```python
from build123d import *

# Parameters (mm, degrees)
BOSS_EXTRU_1_DEPTH           = 3
ESQUISSE26_W                 = 21
ESQUISSE26_H                 = 42
ENL_V_MAT_EXTRU_1_DEPTH      = 4
ESQUISSE21_W                 = 11.4
ESQUISSE21_H                 = 11.4
ENL_V_MAT_EXTRU_3_DEPTH      = 4
D_GAGEMENT_M32_D             = 3.4
D_GAGEMENT_M33_D             = 3.4
ENL_V_MAT_EXTRU_4_DEPTH      = 10
ENL_V_MAT_EXTRU_4_DEPTH_BACK = 4
D_GAGEMENT_M41_D             = 4.5
ESQUISSE40_W                 = 13
ESQUISSE40_H                 = 13
ENL_V_MAT_EXTRU_5_DEPTH      = 4


with BuildPart() as part:
    # Esquisse1 → Boss.-Extru.1 (new body)
    with BuildSketch(Plane.XY):
        with BuildLine():
            Line((-145, 85), (-109.886246, 120.113754))
            Line((-109.886246, 120.113754), (109.886246, 120.113754))
            Line((109.886246, 120.113754), (145, 85))
            Line((145, 85), (145, -85))
            Line((145, -85), (109.886246, -120.113754))
            Line((109.886246, -120.113754), (104.886246, -120.113754))
            ThreePointArc((104.886246, -120.113754), (0, -20), (-104.886246, -120.113754))
            Line((-104.886246, -120.113754), (-109.886246, -120.113754))
            Line((-109.886246, -120.113754), (-145, -85))
            Line((-145, -85), (-145, 85))
        make_face()
    extrude(amount=BOSS_EXTRU_1_DEPTH)

    # Esquisse26 → Enlèv. mat.-Extru.1 (cut, through all)
    with BuildSketch(Plane.XY.offset(3)):
        with Locations((-115, -69.113754)):
            Rectangle(ESQUISSE26_W, ESQUISSE26_H)
        with Locations((-115, 69.113754)):
            Rectangle(ESQUISSE26_W, ESQUISSE26_H)
        with Locations((115, 69.113754)):
            Rectangle(ESQUISSE26_W, ESQUISSE26_H)
        with Locations((115, -69.113754)):
            Rectangle(ESQUISSE26_W, ESQUISSE26_H)
    extrude(amount=-ENL_V_MAT_EXTRU_1_DEPTH, mode=Mode.SUBTRACT)

    # Esquisse21 → Enlèv. mat.-Extru.3 (cut, through all)
    with BuildSketch(Plane.XY.offset(3)):
        with Locations((-139.3, 79.3)):
            Rectangle(ESQUISSE21_W, ESQUISSE21_H)
        with Locations((139.3, 79.3)):
            Rectangle(ESQUISSE21_W, ESQUISSE21_H)
        with Locations((-139.3, -79.3)):
            Rectangle(ESQUISSE21_W, ESQUISSE21_H)
        with Locations((139.3, -79.3)):
            Rectangle(ESQUISSE21_W, ESQUISSE21_H)
    extrude(amount=-ENL_V_MAT_EXTRU_3_DEPTH, mode=Mode.SUBTRACT)

    # Dégagement M32 (through all)
    with Locations(Plane.XY.offset(3)):
        with Locations((-120, 93.313754), (-110, 93.313754), (-120, 44.913754), (-110, 44.913754), (-120, -44.913754), (-110, -44.913754), (-120, -93.313754), (-110, -93.313754), (110, -93.313754), (120, -93.313754), (120, -44.913754), (110, -44.913754), (120, 44.913754), (110, 44.913754), (110, 93.313754), (120, 93.313754)):
            Hole(D_GAGEMENT_M32_D / 2)

    # Dégagement M33 (through all)
    with Locations(Plane.XY.offset(3)):
        with Locations((-90, 111.413754), (0, 111.413754), (90, 111.413754)):
            Hole(D_GAGEMENT_M33_D / 2)

    # Esquisse36 → Enlèv. mat.-Extru.4 (cut, two sides)
    with BuildSketch(Plane.XY.offset(3)) as enl_v_mat_extru_4_sk:
        with BuildLine():
            Line((-100, -6.413754), (-65, -6.413754))
            Line((-65, -6.413754), (-65, 38.586246))
            Line((-65, 38.586246), (-100, 38.586246))
            ThreePointArc((-100, 38.586246), (-122.5, 16.086246), (-100, -6.413754))
        make_face()
        with BuildLine():
            Line((100, -6.413754), (65, -6.413754))
            Line((65, -6.413754), (65, 38.586246))
            Line((65, 38.586246), (100, 38.586246))
            ThreePointArc((100, 38.586246), (122.5, 16.086246), (100, -6.413754))
        make_face()
    extrude(amount=ENL_V_MAT_EXTRU_4_DEPTH, mode=Mode.SUBTRACT)
    extrude(enl_v_mat_extru_4_sk.sketch, amount=-ENL_V_MAT_EXTRU_4_DEPTH_BACK, mode=Mode.SUBTRACT)

    # Dégagement M41 (through all)
    with Locations(Plane(origin=(0, 0, 0), x_dir=(-1, 0, 0), z_dir=(0, 0, -1))):
        with Locations((-139.3, 55), (-139.3, 0), (-139.3, -55), (139.3, 55), (139.3, 0), (139.3, -55)):
            Hole(D_GAGEMENT_M41_D / 2)

    # Esquisse40 → Enlèv. mat.-Extru.5 (cut, through all)
    with BuildSketch(Plane.XY.offset(3)):
        with Locations((-60, 90.713754)):
            Rectangle(ESQUISSE40_W, ESQUISSE40_H)
        with Locations((0, 90.713754)):
            Rectangle(ESQUISSE40_W, ESQUISSE40_H)
        with Locations((60, 90.713754)):
            Rectangle(ESQUISSE40_W, ESQUISSE40_H)
    extrude(amount=-ENL_V_MAT_EXTRU_5_DEPTH, mode=Mode.SUBTRACT)


solid = part.part
```
The model under review builds one solid part; all positions refer to its coordinate system, in mm. A direction names the side the tool comes from. Give positions to 0.01 mm unless a question says otherwise; leave off trailing zeros. Write each loop counter-clockwise with the first axis right and the second up, starting at its lowest first coordinate (ties: lowest second). Pieces come first, ordered by that corner, then holes. Notation, with made-up numbers: (15.25, 87.5) -> (46.25, 87.5) arc R22 cw to (46.25, 102.5) -> close; hole circle Ø2 at (72, 53). An arc over 180 degrees is marked (long way). Answer in a Markdown table with one row per item.
1) Clearance check with flat-ended pins moving along their axes: P1, Ø0.9, axis at x = 138, z = 1, coming from the +Y side; P2, Ø4.5, axis at x = -120, y = -93.31, coming from the -Z side; P3, Ø1.5, axis at x = -141.5, z = 2, coming from the +Y side; P4, Ø0.9, axis at y = 92.5, z = 2, coming from the -X side. State where each tip first meets the part, or that it passes through.
Worked answers:
| item | result |
|---|---|
| P1 | y = 92.45 |
| P2 | z = 0 |
| P3 | y = 89.25 |
| P4 | x = -137.95 |
2) Add section B-B on z = 1.4. Count the separate pieces of the cut face and the enclosed holes in it, plus the area to 3 significant figures.
Worked answers:
| item | result |
|---|---|
| separate pieces | 1 |
| enclosed holes | 34 |
| area | 41,300 mm² |
3) Add section C-C on x = -19. State the section outline as (y, z) points, plus the area to 3 significant figures.
Worked answers:
| item | result |
|---|---|
| outline | (-21.73, 0) -> (120.11, 0) -> (120.11, 3) -> (-21.73, 3) -> close |
| area | 426 mm² |
4) Mouldability with a two-part tool opening along Y and no side actions: class faces 3 (the cylindrical face through (-122.495, 16.581, 1.521)), 4 (the flat face through (2, 28, 3)), 5 (the flat face through (127, 103, 1)), 6 (the flat face through (-127, -103, 1)) as +Y half, -Y half, draft (parallel to the pull), parting line (faces both ways), or undercut.
Worked answers:
| item | result |
|---|---|
| face 3 | undercut |
| face 4 | draft |
| face 5 | +Y half |
| face 6 | -Y half |
5) Add section A-A on x = 60.5. State the section outline as (y, z) points, plus the area to 3 significant figures.
Worked answers:
| item | result |
|---|---|
| outline | (-39.18, 0) -> (84.21, 0) -> (84.21, 3) -> (-39.18, 3) -> close; (97.21, 0) -> (120.11, 0) -> (120.11, 3) -> (97.21, 3) -> close |
| area | 439 mm² |
6) For L1, parallel to X at y = 57.5, z = 2.2; L2, parallel to X at y = -93, z = 0.25 (3 decimals); L3, parallel to X at y = 84.5, z = 0.75, list the stretches that pass through material, from the lowest coordinate up. Write a range as [from, to].
Worked answers:
| item | result |
|---|---|
| L1 | [-145, -125.5], [-104.5, 104.5], [125.5, 145] |
| L2 | [-137, -121.671], [-118.329, -111.671], [-108.329, -100.005], [100.005, 108.329], [111.671, 118.329], [121.671, 137] |
| L3 | [-133.6, -125.5], [-104.5, -66.5], [-53.5, -6.5], [6.5, 53.5], [66.5, 104.5], [125.5, 133.6] |
7) Tool access review of faces 1 (the cylindrical face through (122.495, 16.581, 1.521)), 2 (the flat face through (128, -102, 1)): name each direction out of +Z, -Z, +X, -X, +Y, -Y from which nothing blocks a thin tool from reaching the whole face with its end or side.
Worked answers:
| item | result |
|---|---|
| face 1 | +Z, -Z |
| face 2 | +Z, -Z, +X, -Y |
